from build123d import *

# Parameters (mm, degrees)
SKETCH1_R           = 6.35
SKETCH1_R_2         = 4.7625
BOSS_EXTRUDE1_DEPTH = 3.175
SKETCH1_3_R         = 4.7625
SKETCH1_3_R_2       = 3.475
BOSS_EXTRUDE2_DEPTH = 9.5
CHAMFER1_SIZE       = 3


with BuildPart() as part:
    # Sketch1 → Boss-Extrude1 (new body)
    with BuildSketch(Plane(origin=(0, 0, 0), x_dir=(1, 0, 0), z_dir=(0, 1, 0))):
        with Locations(Location((0, 0, 0), (0, 0, 270))):
            Circle(SKETCH1_R)
        with Locations(Location((0, 0, 0), (0, 0, 270))):
            Circle(SKETCH1_R_2, mode=Mode.SUBTRACT)
    extrude(amount=BOSS_EXTRUDE1_DEPTH)

    # Sketch1<3> → Boss-Extrude2 (add)
    with BuildSketch(Plane(origin=(0, 0, 0), x_dir=(1, 0, 0), z_dir=(0, 1, 0))):
        with Locations(Location((0, 0, 0), (0, 0, 270))):
            Circle(SKETCH1_3_R)
        with Locations(Location((0, 0, 0), (0, 0, 270))):
            Circle(SKETCH1_3_R_2, mode=Mode.SUBTRACT)
    extrude(amount=BOSS_EXTRUDE2_DEPTH)

    # Chamfer1
    # the kernel refuses this chamfer: 3 mm, written as the material it adds along each edge
    with BuildSketch(Plane(origin=(0, 3.175, 0), x_dir=(0, 0, 1), z_dir=(-1, 0, 0))) as chamfer1_piece_1_section:
        Polygon((4.7625 + CHAMFER1_SIZE, 0), (4.7625, CHAMFER1_SIZE), (4.7625, 0), align=None)
    chamfer1_piece_1 = revolve(axis=Axis((0, 3.175, 0), (0, 1, 0)), mode=Mode.PRIVATE)
    chamfer1_piece_1 = chamfer1_piece_1 & Plane(origin=(0, 5.38786909, 0), x_dir=(0, 0, 1), z_dir=(0, -1, 0)) * Cylinder(6.35, 32, mode=Mode.PRIVATE)
    add(chamfer1_piece_1)


solid = part.part
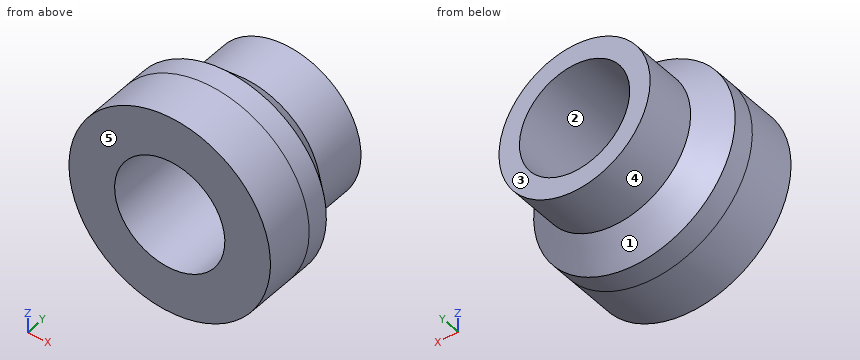
Work out the finished part from the listing and answer in its coordinate system (mm). Face numbers are marked on the shaded views. A direction names the side the tool comes from. Give positions to 0.01 mm unless a question says otherwise; leave off trailing zeros. Loops run counter-clockwise (first coordinate to the right, second up) from the corner with the lowest first, then second, coordinate; pieces in that order, holes last. Notation, with made-up numbers: M -32.5,34 L 6.5,34 A20 cw 6.5,48 Z; hole C -8.75,25 d6. An arc over 180 degrees is marked long. Use CSV: the item, a comma, the result in double quotes.
1) Consider L1, parallel to X at y = 6.25, z = 0 (1 decimal); L2, parallel to X at y = 2, z = 0 (3 decimals); L3, parallel to Z at x = -1, y = 6.5. Determine where each line is inside the solid, lowest interval first.
Answer:
L1,"-4.8 to -3.5, 3.5 to 4.8"
L2,"-6.35 to -3.475, 3.475 to 6.35"
L3,"-4.66 to -3.33, 3.33 to 4.66"
2) Which of the six approach directions +Z, -Z, +X, -X, +Y, -Y give full straight-line access (tool end or side, diameter ignored) to the marked faces 4 and 5?
Answer:
face 4,"+Y"
face 5,"+Z, -Z, +X, -X, -Y"
3) Find section D-D on y = 3.5. Write down the section's boundary in (x, z) (3 decimals).
Answer:
outline,"C 0,0 d12.7; hole C 0,0 d6.95"
4) Given P1, Ø5.5, axis at x = 0, z = 0, coming from the +Y side; P2, Ø5, axis at y = 7, z = -5, coming from the +X side; P3, Ø1, axis at y = 2.5, z = 3, coming from the +X side, each flat-ended and moving along its own axis, determine where each tip first touches the part or whether it passes through.
Answer:
P1,"through"
P2,"x = 4.82"
P3,"x = 5.84"
5) Determine the mould class of the marked faces 1, 2 and 3 for opening direction Z: released by +Z, released by -Z, zero draft, split by the parting line, or undercut.
Answer:
face 1,"split by the parting line"
face 2,"undercut"
face 3,"zero draft"
